from build123d import *

# Parameters (mm, degrees)
F1_R           = 68.35
F2_DEPTH       = 12.7
F4_D           = 9.525
F4_CSINK_D     = 19.8374
F4_CSINK_ANGLE = 82
F6_D           = 6.6
F6_CBORE_D     = 11.25
F6_CBORE_DEPTH = 6


# Not quite as in the source:
# - a length typed as a fraction of an inch, garbled in the dataset ("3 / 203.2 mm" for 3/8 in), is restored
# - a feature names something its author has since deleted; it is built from what else it names


with BuildPart() as f2:
    # F1 (on Top) → F2 (new body)
    with BuildSketch(Plane.XY):
        Circle(F1_R)
    extrude(amount=F2_DEPTH)

    # F4 (through all)
    with Locations(Plane(origin=(0, 0, 0), x_dir=(1, 0, 0), z_dir=(0, 0, -1))):
        with Locations((-39, -39.5575846078), (39, -39.5575846078), (-39, 39.5575846078), (39, 39.5575846078)):
            CounterSinkHole(F4_D / 2, F4_CSINK_D / 2, counter_sink_angle=F4_CSINK_ANGLE)

    # F6 (through all)
    with Locations(Plane.XY.offset(12.7)):
        with Locations((0, 42.5), (42.5, 0), (0, -42.5), (-42.5, 0)):
            CounterBoreHole(F6_D / 2, F6_CBORE_D / 2, F6_CBORE_DEPTH)


solid = f2.part
Verification items for the finished model (mm, model axes). A direction names the side the tool comes from. Coordinates: 2 decimals unless noted, no trailing zeros. Write each loop counter-clockwise with the first axis right and the second up, starting at its lowest first coordinate (ties: lowest second). Pieces come first, ordered by that corner, then holes. Notation, with made-up numbers: M 20.5,47.25 L 65.5,47.25 A35 cw 65.5,81.25 Z; hole C -33,-29.5 d7. An arc over 180 degrees is marked long. Use a Markdown table: item, result.
Q1. Draft check along X on faces 1 (the face through (-1, 1, 0)), 2 (the face through (-54.24, -41.59, 6.26)), 3 (the face through (47.865, 1.69, 9.742)). Enter one of: +X half, -X half, draft (parallel to the pull), parting line (faces both ways), or undercut.
Reply:
| item | result |
|---|---|
| face 1 | draft |
| face 2 | parting line |
| face 3 | undercut |
Q2. Sectioned sample at C-C, the plane z = 4.25. Count the separate pieces of the cut face and the enclosed holes in it, plus the area to 3 significant figures.
Reply:
| item | result |
|---|---|
| separate pieces | 1 |
| enclosed holes | 8 |
| area | 14,100 mm² |
Q3. Sectioned sample at A-A, the plane y = 0. Record the boundary of the cut face in (x, z) (3 decimals).
Reply:
| item | result |
|---|---|
| outline | M -68.35,0 L -45.8,0 L -45.8,6.7 L -48.125,6.7 L -48.125,12.7 L -68.35,12.7 Z; M -39.2,0 L 39.2,0 L 39.2,6.7 L 36.875,6.7 L 36.875,12.7 L -36.875,12.7 L -36.875,6.7 L -39.2,6.7 Z; M 45.8,0 L 68.35,0 L 68.35,12.7 L 48.125,12.7 L 48.125,6.7 L 45.8,6.7 Z |
Q4. Go/stop test with flat-tipped pins: P1, Ø10.5, axis at x = 0, y = -42.5, coming from the +Z side; P2, Ø12.5, axis at x = -39, y = 39.56, coming from the -Z side; P3, Ø15, axis at x = -39, y = -39.56, coming from the -Z side. Record where each tip stops, or that it passes through.
Reply:
| item | result |
|---|---|
| P1 | stops at z = 6.7 |
| P2 | stops at z = 4.22 |
| P3 | stops at z = 2.78 |
Q5. Thickness scan on line 1 (Y direction, x = 42.5, z = 1.75); line 2 (Y direction, x = 42.5, z = 9.95) (3 decimals); line 3 (Z direction, x = 0.5, y = 38.5). Record the ranges inside material, lowest first.
Reply:
| item | result |
|---|---|
| line 1 | y = -53.53 to -47.19, -31.92 to -3.3, 3.3 to 31.92, 47.19 to 53.53 |
| line 2 | y = -53.53 to -42.787, -36.328 to -5.625, 5.625 to 36.328, 42.787 to 53.53 |
| line 3 | z = 0 to 6.7 |
Q6. Set-up check for faces 4 (the face through (-0.732, -36.923, 9.742)), 5 (the face through (36.802, -35.332, 9.363)): record each of +Z, -Z, +X, -X, +Y, -Y from which the full face is reachable in a straight line by a thin tool's end or side.
Reply:
| item | result |
|---|---|
| face 4 | +Z |
| face 5 | +Z, -Z |
